```python
from build123d import *

# Parameters (mm, degrees)
F0_R     = 365.76
F0_R_2   = 111.76
F1_DEPTH = 6.35
F2_W     = 380.011261
F2_H     = 787.612766
F3_DEPTH = 6.351
F5_DEPTH = 6.351
F6_W     = 6.35
F6_H     = 152.4
F7_DEPTH = 76.2
F8_R     = 6.35
F9_DEPTH = 229.281121


with BuildPart() as f1:
    # F0 (on Top) → F1 (new body)
    with BuildSketch(Plane.XY):
        Circle(F0_R)
        Circle(F0_R_2, mode=Mode.SUBTRACT)
    extrude(amount=F1_DEPTH)

    # F2 (on face) → F3 (cut, through all)
    with BuildSketch(Plane.XY.offset(6.35)):
        with Locations((190.00563, 1.120374)):
            Rectangle(F2_W, F2_H)
    extrude(amount=-F3_DEPTH, mode=Mode.SUBTRACT)

    # F4 (on face) → F5 (cut, through all)
    with BuildSketch(Plane.XY.offset(6.35)):
        with BuildLine():
            ThreePointArc((-88.9, 289.56), (-302.899659, 0), (-88.9, -289.56))
            Line((-88.9, -289.56), (-88.9, -264.16))
            ThreePointArc((-88.9, -264.16), (-278.717986, 0), (-88.9, 264.16))
            Line((-88.9, 264.16), (-88.9, 289.56))
        make_face()
        with BuildLine():
            ThreePointArc((-88.9, 187.96), (-207.923475, 0), (-88.9, -187.96))
            Line((-88.9, -187.96), (-88.9, -162.56))
            ThreePointArc((-88.9, -162.56), (-185.28077, 0), (-88.9, 162.56))
            Line((-88.9, 162.56), (-88.9, 187.96))
        make_face()
    extrude(amount=-F5_DEPTH, mode=Mode.SUBTRACT)

    # F6 (on face) → F7 (join)
    with BuildSketch(Plane(origin=(0, 0, 0), x_dir=(1, 0, 0), z_dir=(0, 0, -1))):
        with Locations((-139.654879, 0)):
            Rectangle(F6_W, F6_H)
    extrude(amount=F7_DEPTH)

    # F8 (on face) → F9 (cut, through all)
    with BuildSketch(Plane.YZ.offset(-136.479879)):
        with Locations((0, -38.1)):
            Circle(F8_R)
    extrude(amount=-F9_DEPTH, mode=Mode.SUBTRACT)


solid = f1.part
```
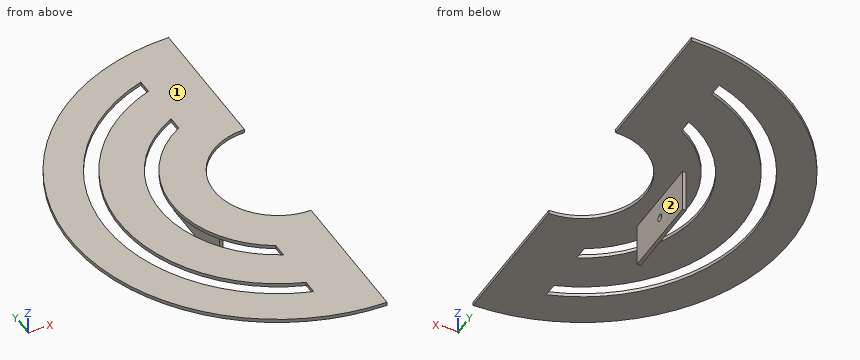
CAD build for the part. Positions are in the model's coordinates, mm. Face numbers are marked on the shaded views. A direction names the side the tool comes from. Round coordinates to 2 decimals unless told otherwise and drop trailing zeros. Write each loop counter-clockwise with the first axis right and the second up, starting at its lowest first coordinate (ties: lowest second). Pieces come first, ordered by that corner, then holes. Notation, with made-up numbers: (6.5, 51.25) -> (13.5, 51.25) arc R26 ccw to (13.5, 70.25) -> close; hole circle Ø11 at (54.5, 43). An arc over 180 degrees is marked (long way). Answer in a Markdown table with one row per item. Add a question column.
Item 1: Drill centre lines: line 1 (X direction, y = -74, z = 1.5); line 2 (Z direction, x = -140.5, y = 0); line 3 (Z direction, x = -108, y = -212). Where is each one in solid material? Low to high. Write a range as from..to.
Item 2: Saw through at C-C, the plane y = -243. Write the cut outline in (x, z).
Item 3: Saw through at D-D, the plane z = -64. Write the cut outline in (x, y), then the cut area to 3 significant figures.
Item 4: Saw through at A-A, the plane y = 150.5. Write the cut outline in (x, z), then the cut area to 3 significant figures.
Item 5: Which spindle directions (+Z, -Z, +X, -X, +Y, -Y) get a long thin tool onto all of the face, cutting with end or side? Do the marked faces 1 and 2. Say none if no direction does.
Item 6: Drop flat-ended pins along their axis: pin 1 Ø5 at (x, z) = (-139.5, -19.5) entering from +Y; pin 2 Ø10 at (y, z) = (0, -38.1) entering from +X; pin 3 Ø23 at (y, z) = (-29.5, -49) entering from +X; pin 4 Ø7 at (y, z) = (-276.5, 2.5) entering from -X. Give the stop position or say it passes through.
Item 7: Saw through at B-B, the plane x = -267. Write the cut outline in (y, z), then the cut area to 3 significant figures.
Findings below:
| question | item | result |
|---|---|---|
| 1 | line 1 | x = -358.2..-293.72, -268.71..-194.31, -169.86..-83.75 |
| 1 | line 2 | z = -76.2..-44.45, -31.75..6.35 |
| 1 | line 3 | z = 0..6.35 |
| 2 | outline | (-273.37, 0) -> (-180.83, 0) -> (-180.83, 6.35) -> (-273.37, 6.35) -> close; (-136.51, 0) -> (0, 0) -> (0, 6.35) -> (-136.51, 6.35) -> close |
| 3 | outline | (-142.83, -76.2) -> (-136.48, -76.2) -> (-136.48, 76.2) -> (-142.83, 76.2) -> close |
| 3 | area | 968 mm^2 |
| 4 | outline | (-333.36, 0) -> (-262.86, 0) -> (-262.86, 6.35) -> (-333.36, 6.35) -> close; (-234.59, 0) -> (-143.46, 0) -> (-143.46, 6.35) -> (-234.59, 6.35) -> close; (-108.07, 0) -> (0, 0) -> (0, 6.35) -> (-108.07, 6.35) -> close |
| 4 | area | 1,710 mm^2 |
| 5 | face 1 | +Z, +X, -X, +Y, -Y |
| 5 | face 2 | -Z, +X, +Y, -Y |
| 6 | pin 1 | stops at y = 76.2 |
| 6 | pin 2 | passes through |
| 6 | pin 3 | stops at x = -136.48 |
| 6 | pin 4 | stops at x = -243.42 |
| 7 | outline | (-249.98, 0) -> (-143.04, 0) -> (-143.04, 6.35) -> (-249.98, 6.35) -> close; (-79.97, 0) -> (79.97, 0) -> (79.97, 6.35) -> (-79.97, 6.35) -> close; (143.04, 0) -> (249.98, 0) -> (249.98, 6.35) -> (143.04, 6.35) -> close |
| 7 | area | 2,370 mm^2 |
